Drawing for the job (mm, zero at the part's lowest x, y, z). Round coordinates to 2 decimals unless told otherwise and drop trailing zeros. Write each loop counter-clockwise with the first axis right and the second up, starting at its lowest first coordinate (ties: lowest second). Pieces come first, ordered by that corner, then holes. Notation, with made-up numbers: M 19,21.25 L 49,21.25 A19 ccw 49,45.25 Z; hole C 5.5,0.25 d2. An arc over 180 degrees is marked long. Use a Markdown table: item, result. Add a question column.
1) Slice it at A-A on z = 1.7. Write the cut outline in (x, y) (1 decimal).
2) Drop a flat-ended pin along its axis: P1, Ø5, axis at x = 193.07, y = 91.41, coming from the -Z side. Give the stop position or say it passes through.
3) Wall check: probe 1 along X at (y, z) = (41, 2.1) (1 decimal); probe 2 along X at (y, z) = (91, 1.4); probe 3 along Y at (x, z) = (192.5, 3.7) (1 decimal). Give the ranges that are in metal, low to high.
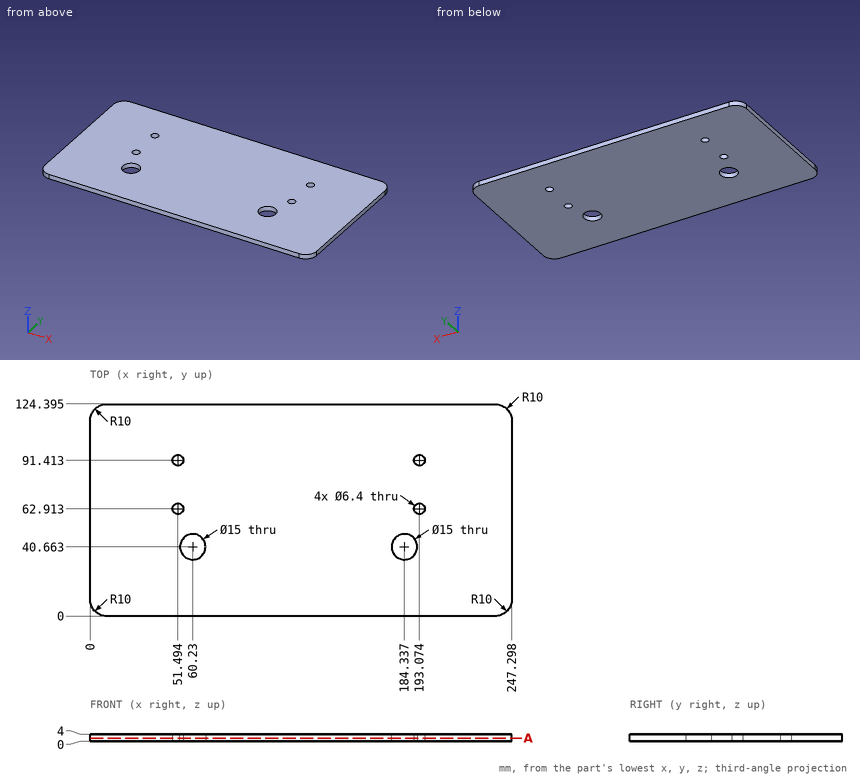
Entries:
| question | item | result |
|---|---|---|
| 1 | outline | M 0,10 A10 ccw 10,0 L 237.3,0 A10 ccw 247.3,10 L 247.3,114.4 A10 ccw 237.3,124.4 L 10,124.4 A10 ccw 0,114.4 Z; hole C 51.5,62.9 d6.4; hole C 51.5,91.4 d6.4; hole C 60.2,40.7 d15; hole C 184.3,40.7 d15; hole C 193.1,62.9 d6.4; hole C 193.1,91.4 d6.4 |
| 2 | P1 | passes through |
| 3 | probe 1 | x = 0 to 52.7, 67.7 to 176.8, 191.8 to 247.3 |
| 3 | probe 2 | x = 0 to 48.32, 54.67 to 189.9, 196.25 to 247.3 |
| 3 | probe 3 | y = 0 to 59.8, 66.1 to 88.3, 94.6 to 124.4 |
